```python
from build123d import *

# Parameters (mm, degrees)
SKETCH1_W           = 41.91
SKETCH1_H           = 63.5
BOSS_EXTRUDE1_DEPTH = 3.175
SKETCH2_W           = 3.175
SKETCH2_H           = 63.5
BOSS_EXTRUDE2_DEPTH = 6.35
SKETCH5_W           = 3.175
SKETCH5_H           = 12.7
BOSS_EXTRUDE4_DEPTH = 16.51
SKETCH6_W           = 9.237604307
SKETCH6_H           = 9.525
SKETCH6_R           = 2.75
BOSS_EXTRUDE5_DEPTH = 6.35
FILLET2_R           = 6.35


with BuildPart() as part:
    # Sketch1 → Boss-Extrude1 (new body)
    with BuildSketch(Plane(origin=(0, 0, 0), x_dir=(1, 0, 0), z_dir=(0, 1, 0))):
        Rectangle(SKETCH1_W, SKETCH1_H)
    extrude(amount=BOSS_EXTRUDE1_DEPTH)

    # Sketch2 → Boss-Extrude2 (add)
    with BuildSketch(Plane(origin=(0, 3.175, 0), x_dir=(1, 0, 0), z_dir=(0, 1, 0))):
        with Locations((-19.3675, 0)):
            Rectangle(SKETCH2_W, SKETCH2_H)
        with Locations((19.3675, 0)):
            Rectangle(SKETCH2_W, SKETCH2_H)
    extrude(amount=BOSS_EXTRUDE2_DEPTH)

    # Sketch5 → Boss-Extrude4 (add)
    with BuildSketch(Plane(origin=(0, 9.525, 0), x_dir=(1, 0, 0), z_dir=(0, 1, 0))):
        with Locations((19.3675, 25.4)):
            Rectangle(SKETCH5_W, SKETCH5_H)
        with Locations((-19.3675, -25.4)):
            Rectangle(SKETCH5_W, SKETCH5_H)
    extrude(amount=BOSS_EXTRUDE4_DEPTH)

    # Sketch6 → Boss-Extrude5 (add)
    # profile 1 of 2: a face of its own
    with BuildSketch(Plane(origin=(0, 26.035, 0), x_dir=(1, 0, 0), z_dir=(0, 1, 0))):
        with Locations((-25.573802154, -26.9875)):
            Rectangle(SKETCH6_W, SKETCH6_H)
        with Locations(Location((-25.573802154, -26.9875, 0), (0, 0, 270))):
            Circle(SKETCH6_R, mode=Mode.SUBTRACT)
    # profile 2 of 2: a face of its own
    with BuildSketch(Plane(origin=(0, 26.035, 0), x_dir=(1, 0, 0), z_dir=(0, 1, 0))):
        with Locations((25.573802154, 26.9875)):
            Rectangle(SKETCH6_W, SKETCH6_H)
        with Locations(Location((25.573802154, 26.9875, 0), (0, 0, 270))):
            Circle(SKETCH6_R, mode=Mode.SUBTRACT)
    extrude(amount=-BOSS_EXTRUDE5_DEPTH)

    # Fillet2
    fillet2_edges = [part.edges().sort_by_distance(p)[0] for p in [
        (19.3675, 9.525, -19.05),
        (-19.3675, 9.525, 19.05),
    ]]
    fillet(fillet2_edges, radius=FILLET2_R)


with BuildPart() as body_2:
    # Mirror1: mirrored copy
    add(part.part.mirror(Plane(origin=(-30.192604307, 19.685, 31.75), x_dir=(0, 0, 1), z_dir=(-1, 0, 0))))


solid = body_2.part
```
Input: part model. Units: mm. Frame: model coordinates. A direction names the side the tool comes from. Give positions to 0.01 mm unless a question says otherwise; leave off trailing zeros. Order: outer loops, then holes, each group sorted by start corner. A loop starts at its lowest first (then second) coordinate and runs counter-clockwise, first axis right, second up.
1. Section D-D on z = -4. Return the cut outline in (x, y) (3 decimals), and give its area (3 significant figures).
Derived:
outline: (-81.34, 0) - (-39.43, 0) - (-39.43, 9.525) - (-42.605, 9.525) - (-42.605, 3.175) - (-78.165, 3.175) - (-78.165, 9.525) - (-81.34, 9.525) - close
area: 173 mm2
2. Pin query (flat end, axial travel): pin 1 (5 mm diameter, centred on x = -84, y = 21.5, fed in from +Z) (3 decimals); pin 2 (7.5 mm diameter, centred on x = -35.5, z = 28, fed in from -Y) (3 decimals); pin 3 (1 mm diameter, centred on x = -41.5, z = -9, fed in from +Y) (3 decimals); pin 4 (3.5 mm diameter, centred on x = -85.96, z = -26.99, fed in from +Y). Return the tip coordinate at first contact, or that it passes through.
Derived:
pin 1: stops at z = -22.225
pin 2: stops at y = 19.685
pin 3: stops at y = 9.525
pin 4: passes through
3. Reachability of faces 1 (the flat face through (-32.7, 19.685, 29)), 2 (the flat face through (-35, 23, 22.225)), 3 (the flat face through (-80, 9.525, 9)), 4 (the flat face through (-87.9, 19.685, -29.2)), 5 (the flat face through (-60, 3.175, 0)) from +Z, -Z, +X, -X, +Y, -Y: full face, straight path, thin tool, end or side. Return the list, or none.
Derived:
face 1: +Z, -Z, +X, -Y
face 2: -Z, +X, +Y, -Y
face 3: +Z, -X, +Y
face 4: +Z, -Z, -X, -Y
face 5: +Z, -Z, +Y
4. Section B-B on z = -27. Return the cut outline in (x, y) (3 decimals), and give its area (3 significant figures).
Derived:
outline: (-90.578, 19.685) - (-88.709, 19.685) - (-88.709, 26.035) - (-90.578, 26.035) - close; (-83.209, 19.685) - (-81.34, 19.685) - (-81.34, 0) - (-39.43, 0) - (-39.43, 9.525) - (-42.605, 9.525) - (-42.605, 3.175) - (-78.165, 3.175) - (-78.165, 26.035) - (-83.209, 26.035) - close
area: 250 mm2
5. Material intervals for L1, parallel to X at y = 5, z = 4; L2, parallel to X at y = 2, z = -11.5; L3, parallel to Y at x = -70.5, z = -13.5 (3 decimals), sorted ascending.
Derived:
L1: x = -81.34 to -78.17, -42.61 to -39.43
L2: x = -81.34 to -39.43
L3: y = 0 to 3.175
6. Mould query, pull axis X, two halves, no side actions, for faces 6 (the flat face through (-42.605, 9, 8)), 7 (the flat face through (-71, 2, -31.75)), 8 (the flat face through (-30.193, 23, 27)). Classes: released by +X, released by -X, zero draft, split by the parting line, or undercut.
Derived:
face 6: undercut
face 7: zero draft
face 8: released by +X
7. Section A-A on y = 18. Return the cut outline in (x, z), and give its area (3 significant figures).
Derived:
outline: (-81.34, -31.75) - (-78.17, -31.75) - (-78.17, -19.05) - (-81.34, -19.05) - close; (-42.61, 19.05) - (-39.43, 19.05) - (-39.43, 31.75) - (-42.61, 31.75) - close
area: 80.6 mm2
8. Section C-C on y = 21.5. Give the number of separate pieces and of enclosed holes in the cut face, and give its area (3 significant figures).
Derived:
separate pieces: 2
enclosed holes: 2
area: 209 mm2
